Check sheet for the drawn part. Datum: minimum x, y, z corner. Units: mm. A direction names the side the tool comes from. Round coordinates to 2 decimals unless told otherwise and drop trailing zeros. Write each loop counter-clockwise with the first axis right and the second up, starting at its lowest first coordinate (ties: lowest second). Pieces come first, ordered by that corner, then holes.
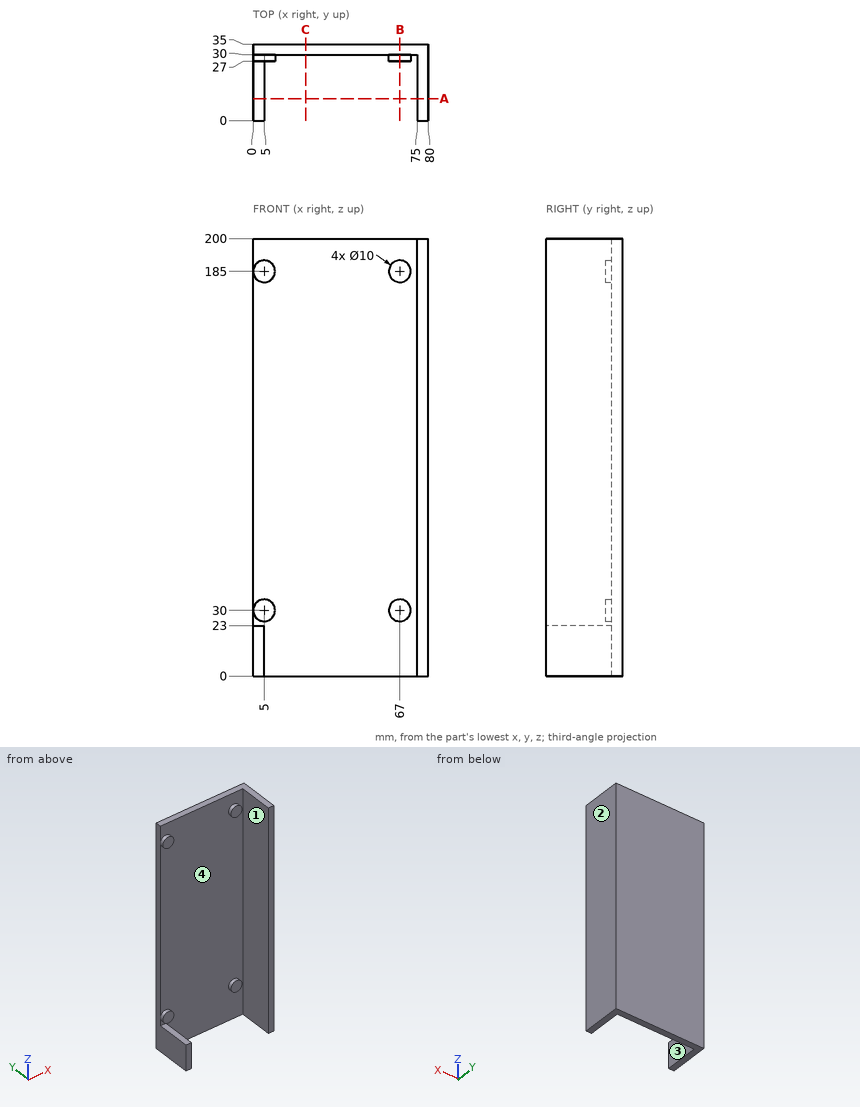
Q1. Depth check by flat-ended pin: P1, Ø3, axis at y = 7.5, z = 94, coming from the -X side; P2, Ø1.5, axis at x = 3.5, y = 19.5, coming from the +Z side; P3, Ø22.5, axis at x = 20.5, z = 85.5, coming from the -Y side. Enter the tip coordinate at first touch or a pass-through.
Recorded:
P1: stops at x = 75
P2: stops at z = 23
P3: stops at y = 30
Q2. Material ranges on line 1 along Y through (x, z) = (23.5, 123.5); line 2 along X through (y, z) = (15, 185.5), recorded low to high.
Recorded:
line 1: y = 30 to 35
line 2: x = 75 to 80
Q3. Tool access check on the marked faces 1 and 2. Record the directions out of +Z, -Z, +X, -X, +Y, -Y that give a thin tool (end or side, any length) a straight path to the whole face; none if there is none.
Recorded:
face 1: +Z, -Z, -Y
face 2: +Z, -Z, +X, +Y, -Y
Q4. Release check for a two-part mould opening along Z. For the marked faces 3 and 4 record: released by +Z, released by -Z, zero draft, split by the parting line, or undercut.
Recorded:
face 3: zero draft
face 4: undercut
Q5. Sectioned sample at A-A (y = 10). Enter the section's corners in (x, z).
Recorded:
outline: (0, 0) - (5, 0) - (5, 23) - (0, 23) - close; (75, 0) - (80, 0) - (80, 200) - (75, 200) - close
Q6. Sectioned sample at B-B (x = 67). Enter the section's corners in (y, z).
Recorded:
outline: (27, 25) - (30, 25) - (30, 0) - (35, 0) - (35, 200) - (30, 200) - (30, 190) - (27, 190) - (27, 180) - (30, 180) - (30, 35) - (27, 35) - close
Q7. Sectioned sample at C-C (x = 24). Enter the section's corners in (y, z).
Recorded:
outline: (30, 0) - (35, 0) - (35, 200) - (30, 200) - close
